The listing builds one solid part. Answer for the finished solid, in the listing's coordinates (mm). A direction names the side the tool comes from. Give positions to 0.01 mm unless a question says otherwise; leave off trailing zeros. Write each loop counter-clockwise with the first axis right and the second up, starting at its lowest first coordinate (ties: lowest second). Pieces come first, ordered by that corner, then holes. Notation, with made-up numbers: (-21.5, 64) -> (3.5, 64) arc R27 cw to (3.5, 91) -> close; hole circle Ø5 at (-34, -24). An arc over 180 degrees is marked (long way). Put each result on its own line as item: value. Start each with the question number.
1) A cutting plane is placed at D-D (x = 3.75). Give the number of separate pieces and of enclosed holes in the cut face, then the cut area to 3 significant figures.
2) For a pull along Y with two mould halves and no side action, classify faces 4 (the flat face through (3, 31.75, -9)), 5 (the flat face through (3, 216, 0)), 6 (the flat face through (3, 260.35, -32)), 7 (the cylindrical face through (3.13, 21.46, -33.6)) as released by +Y, released by -Y, zero draft, split by the parting line, or undercut.
3) A cutting plane is placed at C-C (y = 114). Write down the section's boundary in (x, z), then the cut area to 3 significant figures.
4) A cutting plane is placed at A-A (z = -55). Write down the section's boundary in (x, y), then the cut area to 3 significant figures.
5) For faces 1 (the flat face through (3, 247.65, -54)), 2 (the flat face through (3, 19.05, -13)), 3 (the flat face through (3, 29, 0)), determine the directions among +Z, -Z, +X, -X, +Y, -Y from which every point of the face is accessible in a straight line to the end or side of a thin tool.
6) Flat-ended cylindrical pins translate along their axes: pin 1 Ø1.9 at (x, y) = (4, 23) entering from -Z; pin 2 Ø1.5 at (x, y) = (3.5, 124) entering from -Z. Find the tip coordinate at first contact, or state that the pin passes through.
7) A cutting plane is placed at B-B (z = -23). Write down the section's boundary in (x, y).
8) Find the intervals of material crossed by line 1 along Y through (x, z) = (4, -31.75) (3 decimals); line 2 along Z through (x, y) = (4, 202.35); line 3 along Y through (x, z) = (2.5, -55), in increasing order. Write a range as from..to.
from build123d import *

# Parameters (mm, degrees)
SKETCH1_R           = 2
BOSS_EXTRUDE1_DEPTH = 6.35
SKETCH3_W           = 19.05
SKETCH3_H           = 139.7
CUT_EXTRUDE2_DEPTH  = 6.35
SKETCH2_R           = 1.500000048
SKETCH2_R_2         = 2.5
CUT_EXTRUDE3_DEPTH  = 6.35
SKETCH4_W           = 6.35
SKETCH4_H           = 6.35
CUT_EXTRUDE4_DEPTH  = 6.35
SKETCH5_W           = 19.05
SKETCH5_H           = 6.35
CUT_EXTRUDE5_DEPTH  = 6.35


with BuildPart() as part:
    # Sketch1 → Boss-Extrude1 (new body)
    with BuildSketch(Plane(origin=(0, 0, 0), x_dir=(0, 0, -1), z_dir=(1, 0, 0))):
        Polygon((63.5, 184.15), (63.5, 215.9), (63.5, 228.6), (63.5, 254), (63.5, 260.35), (0, 260.35), (0, 254), (0, 228.6), (0, 215.9), (0, 184.15), (19.05, 184.15), (19.05, 177.8), (0, 177.8), (0, 25.4), (19.05, 25.4), (19.05, 19.05), (0, 19.05), (0, 12.7), (61.867851021, 12.7), (63.5, 12.7), (63.5, 19.05), (57.15, 19.05), (44.45, 19.05), (44.45, 25.4), (57.15, 25.4), (63.5, 25.4), (63.5, 177.8), (44.45, 177.8), (44.45, 184.15), align=None)
        with Locations((31.75, 180.975)):
            Circle(SKETCH1_R, mode=Mode.SUBTRACT)
        with Locations((31.75, 22.225)):
            Circle(SKETCH1_R, mode=Mode.SUBTRACT)
    extrude(amount=BOSS_EXTRUDE1_DEPTH)

    # Sketch3 → Cut-Extrude2 (cut)
    with BuildSketch(Plane(origin=(6.35, 0, 0), x_dir=(0, 0, -1), z_dir=(1, 0, 0))):
        with Locations((9.525, 101.6)):
            Rectangle(SKETCH3_W, SKETCH3_H)
        with Locations((53.975, 101.6)):
            Rectangle(SKETCH3_W, SKETCH3_H)
    extrude(amount=-CUT_EXTRUDE2_DEPTH, mode=Mode.SUBTRACT)

    # Sketch2 → Cut-Extrude3 (cut)
    with BuildSketch(Plane(origin=(6.35, 0, 0), x_dir=(0, 0, -1), z_dir=(1, 0, 0))):
        with Locations((47.250000115, 233.350000152)):
            Circle(SKETCH2_R)
        with Locations((31.75, 217.850000037)):
            Circle(SKETCH2_R_2)
        with Locations((47.250000115, 202.349999922)):
            Circle(SKETCH2_R)
        with Locations((16.249999885, 202.349999922)):
            Circle(SKETCH2_R)
        with Locations((16.249999885, 233.350000152)):
            Circle(SKETCH2_R)
    extrude(amount=-CUT_EXTRUDE3_DEPTH, mode=Mode.SUBTRACT)

    # Sketch4 → Cut-Extrude4 (cut)
    with BuildSketch(Plane(origin=(6.35, 0, 0), x_dir=(0, 0, -1), z_dir=(1, 0, 0))):
        with Locations((22.225, 22.225)):
            Rectangle(SKETCH4_W, SKETCH4_H)
        with Locations((41.275, 22.225)):
            Rectangle(SKETCH4_W, SKETCH4_H)
    extrude(amount=-CUT_EXTRUDE4_DEPTH, mode=Mode.SUBTRACT)

    # Sketch5 → Cut-Extrude5 (cut)
    with BuildSketch(Plane(origin=(6.35, 0, 0), x_dir=(0, 0, -1), z_dir=(1, 0, 0))):
        with Locations((9.525, 250.825)):
            Rectangle(SKETCH5_W, SKETCH5_H)
        with Locations((53.975, 250.825)):
            Rectangle(SKETCH5_W, SKETCH5_H)
    extrude(amount=-CUT_EXTRUDE5_DEPTH, mode=Mode.SUBTRACT)


solid = part.part
Reply:
1. separate pieces: 1
1. enclosed holes: 7
1. area: 9,520 mm2
2. face 4: undercut
2. face 5: zero draft
2. face 6: released by +Y
2. face 7: undercut
3. outline: (0, -44.45) -> (6.35, -44.45) -> (6.35, -19.05) -> (0, -19.05) -> close
3. area: 161 mm2
4. outline: (0, 12.7) -> (6.35, 12.7) -> (6.35, 19.05) -> (0, 19.05) -> close; (0, 25.4) -> (6.35, 25.4) -> (6.35, 31.75) -> (0, 31.75) -> close; (0, 171.45) -> (6.35, 171.45) -> (6.35, 177.8) -> (0, 177.8) -> close; (0, 184.15) -> (6.35, 184.15) -> (6.35, 247.65) -> (0, 247.65) -> close; (0, 254) -> (6.35, 254) -> (6.35, 260.35) -> (0, 260.35) -> close
4. area: 565 mm2
5. face 1: -Z, +X, -X
5. face 2: +Z, +X, -X
5. face 3: +Z, +X, -X, +Y, -Y
6. pin 1: stops at z = -38.1
6. pin 2: stops at z = -44.45
7. outline: (0, 12.7) -> (6.35, 12.7) -> (6.35, 19.05) -> (0, 19.05) -> close; (0, 25.4) -> (6.35, 25.4) -> (6.35, 260.35) -> (0, 260.35) -> close
8. line 1: y = 12.7..20.225, 24.225..178.975, 182.975..215.35, 220.35..260.35
8. line 2: z = -63.5..-48.75, -45.75..-17.75, -14.75..0
8. line 3: y = 12.7..19.05, 25.4..31.75, 171.45..177.8, 184.15..247.65, 254..260.35
